Here's how the part is built. I have some questions about the finished solid (model axes, mm). A direction names the side the tool comes from. Coordinates: 2 decimals unless noted, no trailing zeros. Loops run counter-clockwise (first coordinate to the right, second up) from the corner with the lowest first, then second, coordinate; pieces in that order, holes last.
```python
from build123d import *

# Parameters (mm, degrees)
F1_DEPTH = 5
F2_T     = -1
F3_DEPTH = 5
F5_DEPTH = 5.8358486101
F6_SIZE  = 0.6
F4_W     = 1
F4_H     = 1
F7_DEPTH = 1


with BuildPart() as f1:
    # F0 (on Top) → F1 (new body)
    with BuildSketch(Plane.XY):
        with BuildLine():
            ThreePointArc((0, -5), (-5, 0), (0, 5))
            Line((0, 5), (9.7979589711, 5))
            ThreePointArc((9.7979589711, 5), (-11, 0), (9.7979589711, -5))
            Line((9.7979589711, -5), (0, -5))
        make_face()
        with BuildLine():
            ThreePointArc((0, 5), (3.5355339059, 3.5355339059), (5, 0))
            ThreePointArc((5, 0), (3.5355339059, -3.5355339059), (0, -5))
            Line((0, -5), (9.7979589711, -5))
            ThreePointArc((9.7979589711, -5), (10.695268783, -2.5712303784), (11, 0))
            ThreePointArc((11, 0), (10.695268783, 2.5712303784), (9.7979589711, 5))
            Line((9.7979589711, 5), (0, 5))
        make_face()
    extrude(amount=F1_DEPTH)

    # F2
    f2_openings = [f1.faces().sort_by_distance(p)[0] for p in [
        (-9.520831, 4.858579, 0),
    ]]
    offset(amount=F2_T, openings=f2_openings)

    # F0 (on Top) → F3 (join)
    with BuildSketch(Plane.XY):
        with BuildLine():
            Line((15, 5), (9.7979589711, 5))
            ThreePointArc((9.7979589711, 5), (10.695268783, 2.5712303784), (11, 0))
            ThreePointArc((11, 0), (10.695268783, -2.5712303784), (9.7979589711, -5))
            Line((9.7979589711, -5), (15, -5))
            Line((15, -5), (15, 5))
        make_face()
    extrude(amount=F3_DEPTH)

    # F4 (on face) → F5 (cut, through all)
    with BuildSketch(Plane.YZ.offset(15)):
        Polygon((-4, 2), (-4, 1), (-0.5, 1), (0.5, 1), (4, 1), (4, 2), (4, 3), (4, 4), (0.5, 4), (-0.5, 4), (-4, 4), (-4, 3), align=None)
    extrude(amount=-F5_DEPTH, mode=Mode.SUBTRACT)

    # F6
    f6_edges = [f1.edges().sort_by_distance(p)[0] for p in [
        (-11, 0, 5),
        (0, -5, 5),
    ]]
    chamfer(f6_edges, length=F6_SIZE)

    # F4 (on face) → F7 (cut)
    with BuildSketch(Plane.YZ.offset(15)):
        with Locations((0, 4.5)):
            Rectangle(F4_W, F4_H)
        with Locations((-4.5, 2.5)):
            Rectangle(F4_W, F4_H)
        with Locations((0, 0.5)):
            Rectangle(F4_W, F4_H)
        with Locations((4.5, 2.5)):
            Rectangle(F4_W, F4_H)
    extrude(amount=-F7_DEPTH, mode=Mode.SUBTRACT)


solid = f1.part
```
1. I want a section at A-A (x = 11). Please give me the cut outline in (y, z), then the cut area to 3 significant figures.
2. For pin 1 (0.5 mm diameter, centred on x = 14.5, z = 4.5, fed in from -Y); pin 2 (0.5 mm diameter, centred on x = 14.5, y = -4.5, fed in from -Z); pin 3 (0.5 mm diameter, centred on y = 0, z = 4.5, fed in from +X); pin 4 (2.5 mm diameter, centred on x = 12.5, z = 3, fed in from +Y), each with a flat end and sliding along its axis, tell me the tip position at first contact or that it passes through.
3. I want a section at B-B (y = -1.5). Give the number of separate pieces and of enclosed holes in the cut face, then the cut area to 3 significant figures.
4. We'd pull the mould along X, two halves only. Please class faces 1 (the flat face through (12, -4, 3)), 2 (the flat face through (5, -4, 4)), 3 (the flat face through (15, 3.2, 0.8)), 4 (the cylindrical face through (-11, 0, 2)): +X half, -X half, draft (parallel to the pull), parting line (faces both ways), or undercut.
5. On a 3-axis mill with a long thin cutter (end or side, diameter ignored), from which of +Z, -Z, +X, -X, +Y, -Y can I reach the whole of each face in a straight line? I mean faces 5 (the flat face through (14.5, -4.5, 3)), 6 (the flat face through (12, 4, 2)), 7 (the flat face through (14, 0, 4.5)). Say none if no direction works.
6. I need wall thicknesses on line 1 along X through (y, z) = (0.25, 1.95); line 2 along Y through (x, z) = (0, 1.8); line 3 along Y through (x, z) = (4, 3.7). Which ranges of each line are inside material? Lowest first, please.
Response values:
1. outline: (-5, 0) - (5, 0) - (5, 5) - (-5, 5) - close; hole (-4, 1) - (4, 1) - (4, 4) - (-4, 4) - close
1. area: 26.0 mm2
2. pin 1: stops at y = -5
2. pin 2: stops at z = 0
2. pin 3: stops at x = 14
2. pin 4: stops at y = 5
3. separate pieces: 3
3. enclosed holes: 0
3. area: 33.3 mm2
4. face 1: draft
4. face 2: undercut
4. face 3: +X half
4. face 4: parting line
5. face 5: +X, +Y, -Y
5. face 6: +X
5. face 7: +Z, -Z, +X
6. line 1: x = -11 to -10, -5.99 to -4.99, 4.99 to 5.99
6. line 2: y = -11 to -10, -6 to -5, 5 to 6, 10 to 11
6. line 3: y = -10.25 to -9.17, -4.47 to -3, 3 to 4.47, 9.17 to 10.25
